Input: part model. Units: mm. Frame: model coordinates. A direction names the side the tool comes from. Round coordinates to 2 decimals unless told otherwise and drop trailing zeros. Loops run counter-clockwise (first coordinate to the right, second up) from the corner with the lowest first, then second, coordinate; pieces in that order, holes last. Notation, with made-up numbers: (48.25, 30) -> (105.25, 30) arc R26 ccw to (105.25, 54) -> close; hole circle Ø3 at (20.5, 41.25). An arc over 180 degrees is marked (long way). Answer as a JSON object with one key per item and string values.
```python
from build123d import *

# Parameters (mm, degrees)
F0_W     = 73.025
F0_H     = 44.45
F1_DEPTH = 76.2
F2_W     = 48.26
F2_H     = 38.1
F3_DEPTH = 72.39
F5_DEPTH = 76.2
F6_DEPTH = 76.2


with BuildPart() as f1:
    # F0 (on Top) → F1 (new body)
    with BuildSketch(Plane.XY):
        Rectangle(F0_W, F0_H)
    extrude(amount=F1_DEPTH)

    # F2 (on face) → F3 (cut)
    with BuildSketch(Plane.XY.offset(76.2)):
        Rectangle(F2_W, F2_H)
    extrude(amount=-F3_DEPTH, mode=Mode.SUBTRACT)

    # F4 (on face) → F5 (cut)
    with BuildSketch(Plane.XY.offset(76.2)):
        Polygon((36.5125, -2.54), (36.5125, 0), (36.5125, 2.54), (32.113091, 5.08), (32.113091, -5.08), align=None)
    extrude(amount=-F5_DEPTH, mode=Mode.SUBTRACT)

    # F4 (on face) → F6 (join)
    with BuildSketch(Plane.XY.offset(76.2)):
        Polygon((-36.5125, 0), (-36.5125, 2.54), (-40.911909, 5.08), (-40.911909, -5.08), (-36.5125, -2.54), align=None)
    extrude(amount=-F6_DEPTH)


solid = f1.part
```
1) Ray query, probe 1 along X at (y, z) = (-17.5, 32.5); probe 2 along X at (y, z) = (-2.5, 38.5); probe 3 along Y at (x, z) = (-20.5, 48) (3 decimals). Return the intervals inside material, ascending.
Output:
{"probe 1": "x = -36.51 to -24.13, 24.13 to 36.51", "probe 2": "x = -40.91 to -24.13, 24.13 to 32.11", "probe 3": "y = -22.225 to -19.05, 19.05 to 22.225"}
2) Section B-B, the plane x = -8.5. Output: boundary loops of the cut face in (y, z) (3 decimals).
Output:
{"outline": "(-22.225, 0) -> (22.225, 0) -> (22.225, 76.2) -> (19.05, 76.2) -> (19.05, 3.81) -> (-19.05, 3.81) -> (-19.05, 76.2) -> (-22.225, 76.2) -> close"}
3) Reachability of faces 4 (the face through (0, 19.05, 41)), 5 (the face through (34.344, 3.792, 38.633)), 6 (the face through (-40.912, 0, 39)) from +Z, -Z, +X, -X, +Y, -Y: full face, straight path, thin tool, end or side. Return the list, or none.
Output:
{"face 4": "+Z", "face 5": "+Z, -Z", "face 6": "+Z, -Z, -X, +Y, -Y"}
4) Draft query along Y for faces 1 (the face through (-38.743, -3.828, 38.633)), 2 (the face through (-24.13, 0, 41)), 3 (the face through (-38.68, 3.79, 38.63)). Return one class per face: +Y half, -Y half, draft (parallel to the pull), parting line (faces both ways), or undercut.
Output:
{"face 1": "-Y half", "face 2": "undercut", "face 3": "+Y half"}
5) Section C-C, the plane y = -14.5. Output: boundary loops of the cut face in (x, z).
Output:
{"outline": "(-36.51, 0) -> (36.51, 0) -> (36.51, 76.2) -> (24.13, 76.2) -> (24.13, 3.81) -> (-24.13, 3.81) -> (-24.13, 76.2) -> (-36.51, 76.2) -> close"}
